from build123d import *

# Parameters (mm, degrees)
EXTRUDE_1_DEPTH     = 1.6
CUT_EXTRUDE_START   = 1.6
SKETCH_3_W          = 1.78
SKETCH_3_H          = 8.1
CUT_EXTRUDE_1_DEPTH = 0.1
SKETCH_4_W          = 1.78
SKETCH_4_H          = 8.1
CUT_EXTRUDE_2_DEPTH = 0.1


with BuildPart() as part:
    # 草图1 → 凸台-拉伸1 (new body)
    with BuildSketch(Plane(origin=(0, 0, 0), x_dir=(1, 0, 0), z_dir=(0, 1, 0))):
        with BuildLine():
            Line((11.43, -10), (15, -10))
            Line((15, -10), (15, 10))
            Line((15, 10), (-15, 10))
            Line((-15, 10), (-15, -10))
            Line((-15, -10), (-11.43, -10))
            Line((-11.43, -10), (-11.43, -47.22))
            ThreePointArc((-11.43, -47.22), (-10.990660172, -48.280660172), (-9.93, -48.72))
            Line((-9.93, -48.72), (9.93, -48.72))
            ThreePointArc((9.93, -48.72), (10.990660172, -48.280660172), (11.43, -47.22))
            Line((11.43, -47.22), (11.43, -10))
        make_face()
    extrude(amount=EXTRUDE_1_DEPTH)

    # 草图3 → 切除-拉伸1 (cut)
    with BuildSketch(Plane(origin=(0, 0, 0), x_dir=(1, 0, 0), z_dir=(0, 1, 0)).offset(CUT_EXTRUDE_START)):
        with Locations((-1.275, -44.16)):
            Rectangle(SKETCH_3_W, SKETCH_3_H)
        with Locations((1.275, -44.16)):
            Rectangle(SKETCH_3_W, SKETCH_3_H)
        with Locations((-3.815, -44.16)):
            Rectangle(SKETCH_3_W, SKETCH_3_H)
        with Locations((-6.355, -44.16)):
            Rectangle(SKETCH_3_W, SKETCH_3_H)
        with Locations((-8.895, -44.16)):
            Rectangle(SKETCH_3_W, SKETCH_3_H)
        with Locations((3.815, -44.16)):
            Rectangle(SKETCH_3_W, SKETCH_3_H)
        with Locations((6.355, -44.16)):
            Rectangle(SKETCH_3_W, SKETCH_3_H)
        with Locations((8.895, -44.16)):
            Rectangle(SKETCH_3_W, SKETCH_3_H)
    extrude(amount=-CUT_EXTRUDE_1_DEPTH, mode=Mode.SUBTRACT)

    # 草图4 → 切除-拉伸2 (cut)
    with BuildSketch(Plane(origin=(0, 0, 0), x_dir=(1, 0, 0), z_dir=(0, 1, 0))):
        with Locations((1.275, -44.16)):
            Rectangle(SKETCH_4_W, SKETCH_4_H)
        with Locations((-1.275, -44.16)):
            Rectangle(SKETCH_4_W, SKETCH_4_H)
        with Locations((-8.895, -44.16)):
            Rectangle(SKETCH_4_W, SKETCH_4_H)
        with Locations((-6.355, -44.16)):
            Rectangle(SKETCH_4_W, SKETCH_4_H)
        with Locations((-3.815, -44.16)):
            Rectangle(SKETCH_4_W, SKETCH_4_H)
        with Locations((8.895, -44.16)):
            Rectangle(SKETCH_4_W, SKETCH_4_H)
        with Locations((6.355, -44.16)):
            Rectangle(SKETCH_4_W, SKETCH_4_H)
        with Locations((3.815, -44.16)):
            Rectangle(SKETCH_4_W, SKETCH_4_H)
    extrude(amount=CUT_EXTRUDE_2_DEPTH, mode=Mode.SUBTRACT)


solid = part.part
Geometry check sheet. Reference: the model listing, model coordinates, mm. A direction names the side the tool comes from. Give positions to 0.01 mm unless a question says otherwise; leave off trailing zeros. Order: outer loops, then holes, each group sorted by start corner. A loop starts at its lowest first (then second) coordinate and runs counter-clockwise, first axis right, second up.
1) Gauge pin test, flat ends, axial feed: pin 1 (0.5 mm diameter, centred on x = -8.5, z = 44, fed in from +Y); pin 2 (0.5 mm diameter, centred on x = 1, z = 43, fed in from -Y); pin 3 (1.5 mm diameter, centred on x = 3, z = 20, fed in from -Y). Record the tip position at first contact, or that the pin passes through.
Results are:
pin 1: stops at y = 1.5
pin 2: stops at y = 0.1
pin 3: stops at y = 0
2) Draft check along Z on faces 1 (the flat face through (-15, 1, 0)), 2 (the flat face through (-13, 1, 10)), 3 (the flat face through (0, 1, -10)), 4 (the flat face through (6, 0.1, 44)). Enter one of: released by +Z, released by -Z, zero draft, split by the parting line, or undercut.
Results are:
face 1: zero draft
face 2: released by +Z
face 3: released by -Z
face 4: undercut
3) Cross-section at A-A (y = 0.9). Record the boundary of the cut face in (x, z).
Results are:
outline: (-15, -10) - (15, -10) - (15, 10) - (11.43, 10) - (11.43, 47.22) arc R1.5 ccw to (9.93, 48.72) - (-9.93, 48.72) arc R1.5 ccw to (-11.43, 47.22) - (-11.43, 10) - (-15, 10) - close
4) Cross-section at C-C (z = 17). Record the boundary of the cut face in (x, y), then the cut area to 3 significant figures.
Results are:
outline: (-11.43, 0) - (11.43, 0) - (11.43, 1.6) - (-11.43, 1.6) - close
area: 36.6 mm2
5) Cross-section at B-B (x = -6). Record the boundary of the cut face in (y, z), then the cut area to 3 significant figures.
Results are:
outline: (0, -10) - (1.6, -10) - (1.6, 40.11) - (1.5, 40.11) - (1.5, 48.21) - (1.6, 48.21) - (1.6, 48.72) - (0, 48.72) - (0, 48.21) - (0.1, 48.21) - (0.1, 40.11) - (0, 40.11) - close
area: 92.3 mm2
6) Tool access check on faces 5 (the flat face through (-1, 0.1, 44)), 6 (the flat face through (4, 1.5, 44)), 7 (the flat face through (13, 1, 10)). Record the directions out of +Z, -Z, +X, -X, +Y, -Y that give a thin tool (end or side, any length) a straight path to the whole face; none if there is none.
Results are:
face 5: -Y
face 6: +Y
face 7: +Z, +X, +Y, -Y
7) Material ranges on probe 1 along X at (y, z) = (1.1, 31); probe 2 along Z at (x, y) = (10, 0.8); probe 3 along Y at (x, z) = (4, 43.5), recorded low to high.
Results are:
probe 1: x = -11.43 to 11.43
probe 2: z = -10 to 48.72
probe 3: y = 0.1 to 1.5
